```python
from build123d import *

# Parameters (mm, degrees)
BOSS_EXTRUDE2_DEPTH = 1.5
SKETCH4_R           = 1.35
BOSS_EXTRUDE4_DEPTH = 0.5


with BuildPart() as part:
    # Sketch2 → Boss-Extrude2 (new body)
    with BuildSketch(Plane.XY):
        with BuildLine():
            Line((-2.5, -4.8), (2.5, -4.8))
            ThreePointArc((2.5, -4.8), (7.3, 0), (2.5, 4.8))
            Line((2.5, 4.8), (-2.5, 4.8))
            ThreePointArc((-2.5, 4.8), (-7.3, 0), (-2.5, -4.8))
        make_face()
    extrude(amount=BOSS_EXTRUDE2_DEPTH)

    # Sketch4 → Boss-Extrude4 (add)
    with BuildSketch(Plane(origin=(0, 0, 0), x_dir=(-1, 0, 0), z_dir=(0, 0, -1))):
        with BuildLine():
            Line((-12.5, -2.75), (12.5, -2.75))
            ThreePointArc((12.5, -2.75), (15.25, 0), (12.5, 2.75))
            Line((12.5, 2.75), (-12.5, 2.75))
            ThreePointArc((-12.5, 2.75), (-15.25, 0), (-12.5, -2.75))
        make_face()
        with Locations((-12.5, 0)):
            Circle(SKETCH4_R, mode=Mode.SUBTRACT)
        with Locations((12.5, 0)):
            Circle(SKETCH4_R, mode=Mode.SUBTRACT)
    extrude(amount=BOSS_EXTRUDE4_DEPTH)


solid = part.part
```
Can you work these out from the model? Positions are in its coordinate system, mm. A direction names the side the tool comes from. Give positions to 0.01 mm unless a question says otherwise; leave off trailing zeros. Loops run counter-clockwise (first coordinate to the right, second up) from the corner with the lowest first, then second, coordinate; pieces in that order, holes last. Notation, with made-up numbers: M -24.5,-21.75 L 13.5,-21.75 A8 cw 13.5,-14.75 Z; hole C 42,-7 d11. An arc over 180 degrees is marked long. Use one line per item in the form item = value. Start each with the question number.
(1) On a 3-axis mill with a long thin cutter (end or side, diameter ignored), from which of +Z, -Z, +X, -X, +Y, -Y can I reach the whole of each face in a straight line? I mean faces 5 (the cylindrical face through (-11.15, 0.06, -0.25)), 6 (the flat face through (0, -4, 0)), 7 (the flat face through (0, 4, 0)). Say none if no direction works.
(2) I'm going to push flat-ended pins straight in: P1, Ø1, axis at y = -3.5, z = 0.5, coming from the -X side; P2, Ø1.6, axis at x = -9, y = 0.5, coming from the +Z side; P3, Ø0.6, axis at x = -0.5, y = 4, coming from the -Z side. Where does each tip first touch, or does it pass through?
(3) I want a section at D-D, the plane y = -2. Write out the boundary of the cut face in (x, z), and give its area (3 significant figures).
(4) Please list where these lines run through material, in increasing order: line 1 (Y direction, x = 12.5, z = -0.25); line 2 (Y direction, x = -5, z = -0.1); line 3 (Z direction, x = -7, y = 2.5).
(5) I want a section at C-C, the plane x = 8. Write out the boundary of the cut face in (y, z).
(6) I want a section at A-A, the plane y = 0. Write out the boundary of the cut face in (x, z), and give its area (4 significant figures).
(7) I want a section at B-B, the plane z = 1.1. Write out the boundary of the cut face in (x, y), and give its area (3 significant figures).
(8) Thinking about a two-plate mould opening in X: for faces 1 (the cylindrical face through (7.3, -0.1, 0.7)), 2 (the cylindrical face through (13.85, 0.06, -0.25)), 3 (the cylindrical face through (-7.3, 0.1, 0.7)), 4 (the flat face through (11, 0, 0)), which applies, released by +X, released by -X, zero draft, split by the parting line, or undercut?
Worked out:
q1.face_5 = +Z, -Z
q1.face_6 = -Z, +X, -X, -Y
q1.face_7 = -Z, +X, -X, +Y
q2.P1 = -6.25
q2.P2 = 0
q2.P3 = 0
q3.outline = M -14.39,-0.5 L 14.39,-0.5 L 14.39,0 L 6.86,0 L 6.86,1.5 L -6.86,1.5 L -6.86,0 L -14.39,0 Z
q3.area = 35.0 mm²
q4.line_1 = -2.75 to -1.35, 1.35 to 2.75
q4.line_2 = -2.75 to 2.75
q4.line_3 = -0.5 to 0
q5.outline = M -2.75,-0.5 L 2.75,-0.5 L 2.75,0 L -2.75,0 Z
q6.outline = M -15.25,-0.5 L -13.85,-0.5 L -13.85,0 L -15.25,0 Z; M -11.15,-0.5 L 11.15,-0.5 L 11.15,0 L 7.3,0 L 7.3,1.5 L -7.3,1.5 L -7.3,0 L -11.15,0 Z; M 13.85,-0.5 L 15.25,-0.5 L 15.25,0 L 13.85,0 Z
q6.area = 34.45 mm²
q7.outline = M -2.5,-4.8 L 2.5,-4.8 A4.8 ccw 2.5,4.8 L -2.5,4.8 A4.8 ccw Z
q7.area = 120 mm²
q8.face_1 = released by +X
q8.face_2 = undercut
q8.face_3 = released by -X
q8.face_4 = zero draft
